The listing builds one solid part. Answer for the finished solid, in the listing's coordinates (mm). Face numbers are marked on the shaded views. Coordinates: 2 decimals unless noted, no trailing zeros. Write each loop counter-clockwise with the first axis right and the second up, starting at its lowest first coordinate (ties: lowest second). Pieces come first, ordered by that corner, then holes. Notation, with made-up numbers: M 65,-3 L 109,-3 A4 cw 109,3 Z; hole C 24.5,86 d7. An arc over 180 degrees is marked long. Answer as a JSON object with one key per item and string values. Group by question number.
from build123d import *

# Parameters (mm, degrees)
SKETCH1_R           = 3.175
BOSS_EXTRUDE1_DEPTH = 3.175
SKETCH2_R           = 1.7859375
CUT_EXTRUDE1_DEPTH  = 4.175
FILLET1_R           = 2.54


with BuildPart() as part:
    # Sketch1 → Boss-Extrude1 (new body)
    with BuildSketch(Plane(origin=(0, 0, 0), x_dir=(1, 0, 0), z_dir=(0, 1, 0))):
        with BuildLine():
            Line((-14.79629089, 14.647069703), (-5.630860593, -2.935286864))
            ThreePointArc((-5.630860593, -2.935286864), (0.476542645, -6.332093422), (6.006756757, -2.059459459))
            Line((6.006756757, -2.059459459), (12.185135135, 15.960810811))
            ThreePointArc((12.185135135, 15.960810811), (12.570402125, 17.484099646), (12.7, 19.05))
            Line((12.7, 19.05), (12.7, 31.75))
            Line((12.7, 31.75), (-15.875, 31.75))
            Line((-15.875, 31.75), (-15.875, 19.05))
            ThreePointArc((-15.875, 19.05), (-15.601393023, 16.783427227), (-14.79629089, 14.647069703))
        make_face()
        Circle(SKETCH1_R, mode=Mode.SUBTRACT)
    extrude(amount=BOSS_EXTRUDE1_DEPTH)

    # Sketch2 → Cut-Extrude1 (cut, through all)
    with BuildSketch(Plane(origin=(0, 3.175, 0), x_dir=(1, 0, 0), z_dir=(0, 1, 0))):
        with Locations((-12.6875, 18.65)):
            Circle(SKETCH2_R)
        with Locations((9.5125, 28.95)):
            Circle(SKETCH2_R)
    extrude(amount=-CUT_EXTRUDE1_DEPTH, mode=Mode.SUBTRACT)

    # Fillet1
    fillet1_edges = [part.edges().sort_by_distance(p)[0] for p in [
        (-15.875, 1.5875, -31.75),
        (12.7, 1.5875, -31.75),
    ]]
    fillet(fillet1_edges, radius=FILLET1_R)


solid = part.part
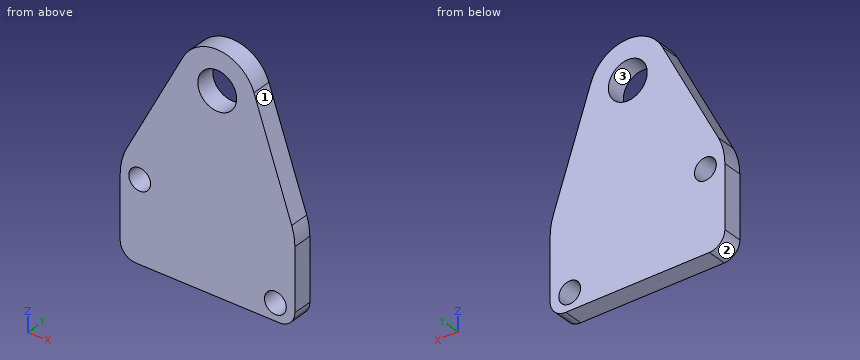
Item 1: For a pull along Z with two mould halves and no side action, classify the marked faces 1, 2 and 3 as +Z half, -Z half, draft (parallel to the pull), parting line (faces both ways), or undercut.
Item 2: A cutting plane is placed at C-C, the plane y = 2. State how many separate pieces and enclosed holes the cut face has, and give its area (3 significant figures).
Item 3: Consider L1, parallel to Z at x = 0, y = 2.4 (3 decimals); L2, parallel to X at y = 2.05, z = -28.95 (3 decimals); L3, parallel to X at y = 1.3, z = -18.65. Determine where each line is inside the solid, lowest interval first. Write a range as from..to.
Item 4: A cutting plane is placed at B-B, the plane z = -18.65. Write down the section's boundary in (x, y) (3 decimals), and give its area (3 significant figures).
Item 5: A cutting plane is placed at D-D, the plane x = 6.5. Write down the section's boundary in (y, z) (3 decimals), and give its area (3 significant figures).
Item 6: Flat-ended cylindrical pins translate along their axes: pin 1 Ø2 at (x, z) = (-12.69, -18.65) entering from -Y; pin 2 Ø1 at (x, y) = (-7, 2) entering from +Z. Find the tip coordinate at first contact, or state that the pin passes through.
Item 7: A cutting plane is placed at A-A, the plane x = 0. Write down the section's boundary in (y, z) (3 decimals).
Answer:
{
 "1": {"face 1": "+Z half", "face 2": "-Z half", "face 3": "undercut"},
 "2": {"separate pieces": "1", "enclosed holes": "3", "area": "792 mm2"},
 "3": {"L1": "-31.75..-3.175, 3.175..6.35", "L2": "-15.875..7.727, 11.298..12.7", "L3": "-15.87..-14.47, -10.9..12.69"},
 "4": {"outline": "M -15.867,0 L -14.473,0 L -14.473,3.175 L -15.867,3.175 Z; M -10.902,0 L 12.692,0 L 12.692,3.175 L -10.902,3.175 Z", "area": "79.3 mm2"},
 "5": {"outline": "M 0,-31.75 L 3.175,-31.75 L 3.175,0.621 L 0,0.621 Z", "area": "103 mm2"},
 "6": {"pin 1": "through", "pin 2": "z = 1.27"},
 "7": {"outline": "M 0,-31.75 L 3.175,-31.75 L 3.175,-3.175 L 0,-3.175 Z; M 0,3.175 L 3.175,3.175 L 3.175,6.35 L 0,6.35 Z"}
}
